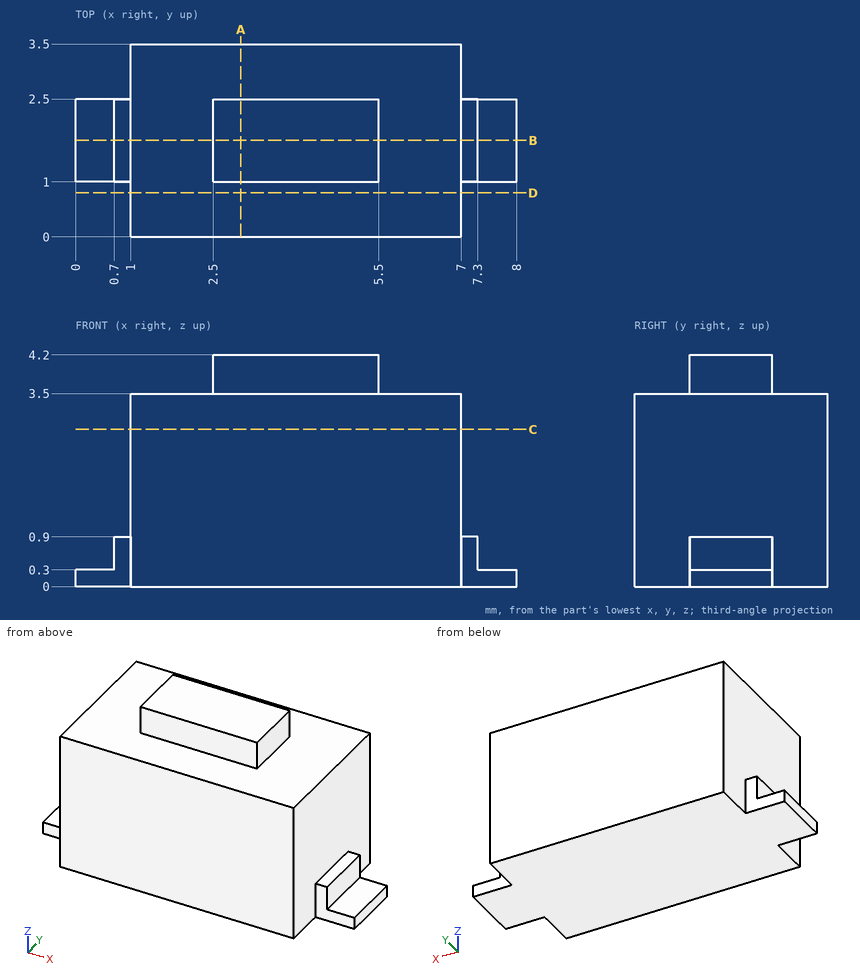
The drawing under review shows one solid part. Ordinate dimensions are in mm from its lowest x, y, z. Give positions to 0.01 mm unless a question says otherwise; leave off trailing zeros. Write each loop counter-clockwise with the first axis right and the second up, starting at its lowest first coordinate (ties: lowest second). Pieces come first, ordered by that corner, then holes.
1. Add section C-C, the plane z = 2.85. Write out the cut boundary in (x, y).
2. Wall thickness on L1, parallel to Z at x = 6, y = 3.3; L2, parallel to X at y = 1.95, z = 1.1; L3, parallel to X at y = 1.5, z = 3.65: over which ranges is each line inside the solid? List them lowest first.
3. For P1, Ø0.8, axis at y = 2, z = 3.5, coming from the +X side; P2, Ø0.8, axis at x = 0.5, y = 1.5, coming from the +Z side; P3, Ø0.8, axis at y = 2, z = 4, coming from the -X side, all flat-tipped, find the tip position at first contact; note any pin that passes through.
4. Add section B-B, the plane y = 1.75. Write out the cut boundary in (x, z).
5. Add section A-A, the plane x = 3. Write out the cut boundary in (y, z).
Worked answers:
1. outline: (1, 0) - (7, 0) - (7, 3.5) - (1, 3.5) - close
2. L1: z = 0 to 3.5
2. L2: x = 1 to 7
2. L3: x = 2.5 to 5.5
3. P1: stops at x = 7
3. P2: stops at z = 0.9
3. P3: stops at x = 2.5
4. outline: (0, 0) - (8, 0) - (8, 0.3) - (7.3, 0.3) - (7.3, 0.9) - (7, 0.9) - (7, 3.5) - (5.5, 3.5) - (5.5, 4.2) - (2.5, 4.2) - (2.5, 3.5) - (1, 3.5) - (1, 0.9) - (0.7, 0.9) - (0.7, 0.3) - (0, 0.3) - close
5. outline: (0, 0) - (3.5, 0) - (3.5, 3.5) - (2.5, 3.5) - (2.5, 4.2) - (1, 4.2) - (1, 3.5) - (0, 3.5) - close
